Could you check a few things on this model? Use its own coordinates, in mm. A direction names the side the tool comes from. Give positions to 0.01 mm unless a question says otherwise; leave off trailing zeros. Order: outer loops, then holes, each group sorted by start corner. A loop starts at its lowest first (then second) coordinate and runs counter-clockwise, first axis right, second up.
(1) If we mould it in two halves opening along X, with no side actions, what happens to faces 6 (the cylindrical face through (-34.531, 3.521, -33.156)), 7 (the flat face through (-1, 0, 3)), 8 (the flat face through (50, 4, 40)), 9 (the flat face through (-1, 31, 146.95))? For each: released by +X, released by -X, zero draft, split by the parting line, or undercut.
(2) If I drill on probe 1 along X at (y, z) = (1.35, -36.95); probe 2 along Z at (x, y) = (-37, 31); probe 3 along Z at (x, y) = (36.95, 4.1), over which ranges is the centre line in solid material (lowest first)?
(3) Imagine slicing it at B-B, the plane z = 130. Write out the boundary of the cut face in (x, y).
(4) On a 3-axis mill with a long thin cutter (end or side, diameter ignored), from which of +Z, -Z, +X, -X, +Y, -Y can I reach the whole of each face in a straight line? I mean faces 1 (the flat face through (-1, 20, 50)), 2 (the flat face through (65, 31, 106.95)), 3 (the flat face through (-35, 2, 35)), 4 (the flat face through (-1, 27, 162)), 5 (the flat face through (-65, 31, 106.95)). Say none if no direction works.
(5) Imagine slicing it at D-D, the plane z = 203. Write out the boundary of the cut face in (x, y), then the cut area to 3 significant figures.
(6) Will these pins go through, and if not, where does the flat tip stop? pin 1 (4 mm diameter, centred on x = -62, y = 32.5, fed in from -Z); pin 2 (4 mm diameter, centred on x = 33, y = 32, fed in from -Z); pin 3 (3 mm diameter, centred on x = -49.5, y = 14, fed in from +Z); pin 4 (4.5 mm diameter, centred on x = 36.95, z = -36.95, fed in from -Y).
(7) Imagine slicing it at C-C, the plane x = -22. Write out the boundary of the cut face in (y, z).
(8) Imagine slicing it at A-A, the plane x = -64. Write out the boundary of the cut face in (y, z), then the cut area to 3 significant figures.
from build123d import *

# Parameters (mm, degrees)
SKETCH1_W           = 100
SKETCH1_H           = 100
SKETCH1_R           = 2.5
BOSS_EXTRUDE1_DEPTH = 5
CUT_EXTRUDE1_START  = -5
SKETCH6_R           = 4.5
CUT_EXTRUDE1_DEPTH  = 3
SKETCH8_W           = 8
SKETCH8_H           = 35
BOSS_EXTRUDE2_DEPTH = 100
SKETCH9_W           = 100
SKETCH9_H           = 8
BOSS_EXTRUDE3_DEPTH = 210
SKETCH10_W          = 160
SKETCH10_H          = 50
BOSS_EXTRUDE4_DEPTH = 8
SKETCH11_W          = 140
SKETCH11_H          = 30
CUT_EXTRUDE2_DEPTH  = 8
SKETCH13_R          = 1
CUT_EXTRUDE3_DEPTH  = 8


with BuildPart() as part:
    # Sketch1 → Boss-Extrude1 (new body)
    with BuildSketch(Plane(origin=(0, 0, 0), x_dir=(1, 0, 0), z_dir=(0, 1, 0))):
        Rectangle(SKETCH1_W, SKETCH1_H)
        with Locations((-36.95, 36.95)):
            Circle(SKETCH1_R, mode=Mode.SUBTRACT)
        with Locations((36.95, 36.95)):
            Circle(SKETCH1_R, mode=Mode.SUBTRACT)
        with Locations((36.95, -36.95)):
            Circle(SKETCH1_R, mode=Mode.SUBTRACT)
        with Locations((-36.95, -36.95)):
            Circle(SKETCH1_R, mode=Mode.SUBTRACT)
    extrude(amount=BOSS_EXTRUDE1_DEPTH)

    # Sketch6 → Cut-Extrude1 (cut)
    with BuildSketch(Plane.XZ.offset(CUT_EXTRUDE1_START)):
        with Locations((-36.95, 36.95)):
            Circle(SKETCH6_R)
        with Locations((36.95, 36.95)):
            Circle(SKETCH6_R)
        with Locations((36.95, -36.95)):
            Circle(SKETCH6_R)
        with Locations((-36.95, -36.95)):
            Circle(SKETCH6_R)
    extrude(amount=CUT_EXTRUDE1_DEPTH, mode=Mode.SUBTRACT)

    # Sketch8 → Boss-Extrude2 (add, through all)
    with BuildSketch(Plane.ZY.offset(50)):
        with Locations((54, 17.5)):
            Rectangle(SKETCH8_W, SKETCH8_H)
    extrude(amount=-BOSS_EXTRUDE2_DEPTH)

    # Sketch9 → Boss-Extrude3 (add)
    with BuildSketch(Plane.XY.offset(58)):
        with Locations((0, 31)):
            Rectangle(SKETCH9_W, SKETCH9_H)
    extrude(amount=BOSS_EXTRUDE3_DEPTH)

    # Sketch10 → Boss-Extrude4 (add)
    with BuildSketch(Plane(origin=(0, 35, 0), x_dir=(1, 0, 0), z_dir=(0, 1, 0))):
        with Locations((0, -131.95)):
            Rectangle(SKETCH10_W, SKETCH10_H)
    extrude(amount=-BOSS_EXTRUDE4_DEPTH)

    # Sketch11 → Cut-Extrude2 (cut)
    with BuildSketch(Plane(origin=(0, 35, 0), x_dir=(1, 0, 0), z_dir=(0, 1, 0))):
        with Locations((0, -131.95)):
            Rectangle(SKETCH11_W, SKETCH11_H)
    extrude(amount=-CUT_EXTRUDE2_DEPTH, mode=Mode.SUBTRACT)

    # Sketch13 → Cut-Extrude3 (cut)
    with BuildSketch(Plane(origin=(0, 35, 0), x_dir=(1, 0, 0), z_dir=(0, 1, 0))):
        with Locations((-37, -181)):
            Circle(SKETCH13_R)
        with Locations((37, -181)):
            Circle(SKETCH13_R)
        with Locations((37, -255)):
            Circle(SKETCH13_R)
        with Locations((-37, -255)):
            Circle(SKETCH13_R)
    extrude(amount=-CUT_EXTRUDE3_DEPTH, mode=Mode.SUBTRACT)


solid = part.part
Answer block:
1. face 6: undercut
1. face 7: zero draft
1. face 8: released by +X
1. face 9: undercut
2. probe 1: x = -50 to -39.45, -34.45 to 34.45, 39.45 to 50
2. probe 2: z = 50 to 116.95, 146.95 to 180, 182 to 254, 256 to 268
2. probe 3: z = -50 to -41.45, -32.45 to 32.45, 41.45 to 58
3. outline: (-80, 27) - (-70, 27) - (-70, 35) - (-80, 35) - close; (70, 27) - (80, 27) - (80, 35) - (70, 35) - close
4. face 1: -Z, +X, -X, +Y
4. face 2: -Z, +X, +Y, -Y
4. face 3: +Y
4. face 4: +Z, +X, -X, -Y
4. face 5: -Z, -X, +Y, -Y
5. outline: (-50, 27) - (50, 27) - (50, 35) - (-50, 35) - close
5. area: 800 mm2
6. pin 1: stops at z = 106.95
6. pin 2: stops at z = 50
6. pin 3: stops at z = 58
6. pin 4: passes through
7. outline: (0, -50) - (5, -50) - (5, 50) - (35, 50) - (35, 116.95) - (27, 116.95) - (27, 58) - (0, 58) - close; (27, 146.95) - (35, 146.95) - (35, 268) - (27, 268) - close
8. outline: (27, 106.95) - (35, 106.95) - (35, 116.95) - (27, 116.95) - close; (27, 146.95) - (35, 146.95) - (35, 156.95) - (27, 156.95) - close
8. area: 160 mm2
